CAD build for the part. Positions are in the model's coordinates, mm. A direction names the side the tool comes from. Coordinates: 2 decimals unless noted, no trailing zeros. Order: outer loops, then holes, each group sorted by start corner. A loop starts at its lowest first (then second) coordinate and runs counter-clockwise, first axis right, second up. Notation, with made-up numbers: M -32.75,-38 L 10.25,-38 A23 ccw 10.25,-15 Z; hole C 37.25,17.25 d9. An arc over 180 degrees is marked long. Write item = value, one per line.
from build123d import *

# Parameters (mm, degrees)
F0_R     = 12.5
F1_DEPTH = 4
F2_R     = 0.5
F3_DEPTH = 8
F6_DEPTH = 3


# Not quite as in the source:
# - a fillet or chamfer that OpenCascade refuses, or shapes differently, is made with other operations: its cross-section is extruded or revolved along the edge and cut away or added


with BuildPart() as f1:
    # F0 (on Top) → F1 (new body)
    with BuildSketch(Plane.XY):
        Circle(F0_R)
        with BuildLine():
            Line((-2.2, -2.3237900077), (-2.2, 2.3237900077))
            ThreePointArc((-2.2, 2.3237900077), (3.2, 0), (-2.2, -2.3237900077))
        make_face(mode=Mode.SUBTRACT)
    extrude(amount=F1_DEPTH)

    # F2 (on face) → F3 (join)
    with BuildSketch(Plane.XY.offset(4)):
        with BuildLine():
            Line((-4.5, 6), (-12.5, 0))
            Line((-12.5, 0), (-4.5, -6))
            Line((-4.5, -6), (10.9658560997, -6))
            ThreePointArc((10.9658560997, -6), (12.1103922572, -3.0965140685), (12.5, 0))
            ThreePointArc((12.5, 0), (12.1103922572, 3.0965140685), (10.9658560997, 6))
            Line((10.9658560997, 6), (-4.5, 6))
        make_face()
        Circle(F2_R, mode=Mode.SUBTRACT)
    extrude(amount=F3_DEPTH)

    # F4: chamfer of 10 x 2.6794919243 on 1 edges, made by hand


with BuildPart() as f4_tool2:
    # F4_s3 → F4_t4 (revolve)
    with BuildSketch(Plane.XZ):
        Polygon((3.1794919243, 4), (0.5, 14), (0.5, 4), align=None)
    revolve(axis=Axis((0, 0, 4), (0, 0, 1)))

    split(bisect_by=Plane.YZ.offset(-2.2), keep=Keep.TOP)


with BuildPart() as f1_1:
    add(f1.part)

    # F4_t1: cut F4_tool2
    add(f4_tool2.part, mode=Mode.SUBTRACT)

    # F5 (on face) → F6 (join)
    with BuildSketch(Plane.XY.offset(12)):
        with BuildLine():
            Line((-4.5, 6), (-12.5, 0))
            Line((-12.5, 0), (-4.5, -6))
            Line((-4.5, -6), (10.9658560997, -6))
            ThreePointArc((10.9658560997, -6), (12.5, 0), (10.9658560997, 6))
            Line((10.9658560997, 6), (-4.5, 6))
        make_face()
    extrude(amount=F6_DEPTH)


solid = f1_1.part
(1) Slice it at C-C, the plane z = 5.5. Write the cut outline in (x, y).
Evaluation:
outline = M -12.5,0 L -4.5,-6 L 10.97,-6 A12.5 ccw 10.97,6 L -4.5,6 Z; hole M -2.2,-1.7 A2.78 ccw long -2.2,1.7 Z
(2) Wall check: line 1 (Y direction, x = 0, z = 1.1); line 2 (X direction, y = 0, z = 2.3); line 3 (Z direction, x = 3.25, y = 7.5). Give the ranges that are in metal, low to high. Write a range as from..to.
Evaluation:
line_1 = -12.5..-3.2, 3.2..12.5
line_2 = -12.5..-2.2, 3.2..12.5
line_3 = 0..4
(3) Tool access for faces 1 (the face through (0, 0, 12)), 2 (the face through (3, 6, 9)), 3 (the face through (-1, -8, 4)), 4 (the face through (-1, 8, 4)): list every direction of +Z, -Z, +X, -X, +Y, -Y with a clear straight run to the whole face (end or side of a thin tool).
Evaluation:
face_1 = -Z
face_2 = +Z, +X, -X, +Y
face_3 = +Z, -X, -Y
face_4 = +Z, -X, +Y
(4) Pull direction Y, two halves, no side cores. Call faces 5 (the face through (-8.556, -2.958, 9.423)), 6 (the face through (-8.444, 3.042, 9.423)), 7 (the face through (1.77, 0.56, 8.94)), 8 (the face through (3, 0, 15)): +Y half, -Y half, draft (parallel to the pull), parting line (faces both ways), or undercut.
Evaluation:
face_5 = -Y half
face_6 = +Y half
face_7 = undercut
face_8 = draft
(5) Pin check, flat tips, straight feed: pin 1 Ø5.5 at (x, z) = (1.5, 12) entering from +Y; pin 2 Ø4 at (y, z) = (-7.5, 4.5) entering from -X; pin 3 Ø3 at (x, z) = (2, 5) entering from +Y. Stop position of each tip, or through.
Evaluation:
pin_1 = 6
pin_2 = -11.19
pin_3 = 12.47
(6) Slice it at D-D, the plane x = -6.5. Write the cut outline in (y, z), then the cut area to 3 significant figures.
Evaluation:
outline = M -10.68,0 L 10.68,0 L 10.68,4 L 4.5,4 L 4.5,15 L -4.5,15 L -4.5,4 L -10.68,4 Z
area = 184 mm²
(7) Slice it at B-B, the plane y = -5.25. Write the cut outline in (x, z).
Evaluation:
outline = M -11.34,0 L 11.34,0 L 11.34,15 L -5.5,15 L -5.5,4 L -11.34,4 Z
